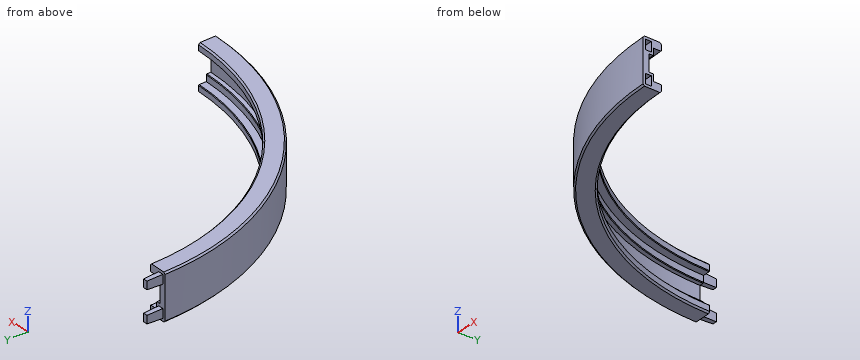
```python
from build123d import *

# Parameters (mm, degrees)
CHANFREIN1_SIZE         = 1
CHANFREIN3_SIZE         = 0.4
ESQUISSE5_W             = 6.3
ESQUISSE5_H             = 3.8
ENL_V_MAT_EXTRU_1_DEPTH = 11
ENL_V_MAT_EXTRU_1_TAPER = 2
ESQUISSE6_W             = 3.4
ESQUISSE6_H             = 5.9
BOSS_EXTRU_2_DEPTH      = 10
BOSS_EXTRU_2_TAPER      = 2


with BuildPart() as part:
    # Balayage1: sweep along a path in Esquisse1
    with BuildLine(Plane.XY) as balayage1_path:
        ThreePointArc((0, 0), (-112.53953952, 46.615403572), (-159.154943092, 159.154943092))
    # Esquisse2 → Balayage1 (sweep)
    with BuildSketch(Plane(origin=(0, 0, 0), x_dir=(0, 0, -1), z_dir=(1, 0, 0))):
        Polygon((-5.5, 0), (5.5, 0), (5.5, 3), (10, 3), (10, 8), (15, 8), (15, -4), (-15, -4), (-15, 8), (-10, 8), (-10, 3), (-5.5, 3), align=None)
    sweep(path=balayage1_path.line)

    # Chanfrein1
    chanfrein1_edges = [part.edges().sort_by_distance(p)[0] for p in [
        (-106.88268527, 52.272257822, 15),
        (-115.367966644, 43.786976448, 15),
        (-115.367966644, 43.786976448, -15),
        (-106.88268527, 52.272257822, -15),
    ]]
    chamfer(chanfrein1_edges, length=CHANFREIN1_SIZE)

    # Chanfrein3
    chanfrein3_edges = [part.edges().sort_by_distance(p)[0] for p in [
        (-106.88268527, 52.272257822, 10),
        (-106.88268527, 52.272257822, -10),
        (-110.418219176, 48.736723916, -5.5),
        (-110.418219176, 48.736723916, 5.5),
    ]]
    chamfer(chanfrein3_edges, length=CHANFREIN3_SIZE)

    # Esquisse5 → Enlèv. mat.-Extru.1 (cut)
    with BuildSketch(Plane(origin=(0, 0, 0), x_dir=(0, 0, -1), z_dir=(1, 0, 0))):
        with Locations((-10.25, -0.5)):
            Rectangle(ESQUISSE5_W, ESQUISSE5_H)
        with Locations((10.25, -0.5)):
            Rectangle(ESQUISSE5_W, ESQUISSE5_H)
    extrude(amount=-ENL_V_MAT_EXTRU_1_DEPTH, taper=ENL_V_MAT_EXTRU_1_TAPER, mode=Mode.SUBTRACT)

    # Esquisse6 → Boss.-Extru.2 (add)
    with BuildSketch(Plane(origin=(0, 159.154943092, 0), x_dir=(1, 0, 0), z_dir=(0, 1, 0))):
        with Locations((-159.654943092, -10.25)):
            Rectangle(ESQUISSE6_W, ESQUISSE6_H)
        with Locations((-159.654943092, 10.25)):
            Rectangle(ESQUISSE6_W, ESQUISSE6_H)
    extrude(amount=BOSS_EXTRU_2_DEPTH, taper=BOSS_EXTRU_2_TAPER)


solid = part.part
```
For this review, take the finished solid that the model builds, in its own axes (mm). Coordinates: 2 decimals unless noted, no trailing zeros. Loops run counter-clockwise (first coordinate to the right, second up) from the corner with the lowest first, then second, coordinate; pieces in that order, holes last. Notation, with made-up numbers: (38, 67.5) - (43, 67.5) arc R19 ccw to (43, 85.5) - close; hole circle Ø8 at (25, 68). An arc over 180 degrees is marked (long way). Use one line per item in the form item = value. Start each with the question number.
1) Take a section at A-A (z = 0.5). State the section outline as (x, y) points, plus the area to 3 significant figures.
2) For pin 1 (12 mm diameter, centred on x = -135.5, y = 105.5, fed in from -Z); pin 2 (0.9 mm diameter, centred on y = -0.5, z = -10, fed in from +X); pin 3 (2 mm diameter, centred on y = 24.5, z = 2, fed in from +X); pin 4 (3.5 mm diameter, centred on x = -160, z = 6, fed in from +Y), all flat-tipped, find the tip position at first contact; note any pin that passes through.
3) To check wall thickness, follow probe 1 along Y at (x, z) = (-7, 13.75); probe 2 along X at (y, z) = (73.5, -7.25); probe 3 along Y at (x, z) = (-60.5, 2.25). State the ranges of each line that lie inside material, in increasing order. Write a range as from..to.
From the geometry:
q1.outline = (-163.15, 159.15) arc R163.15 ccw to (0, -4) - (0, 0) arc R159.15 cw to (-159.15, 159.15) - close
q1.area = 1,010 mm2
q2.pin_1 = -14.58
q2.pin_2 = -11
q2.pin_3 = -83.23
q2.pin_4 = 169.15
q3.probe_1 = -3.85..8.16
q3.probe_2 = -138.86..-130.57
q3.probe_3 = 7.63..11.95
